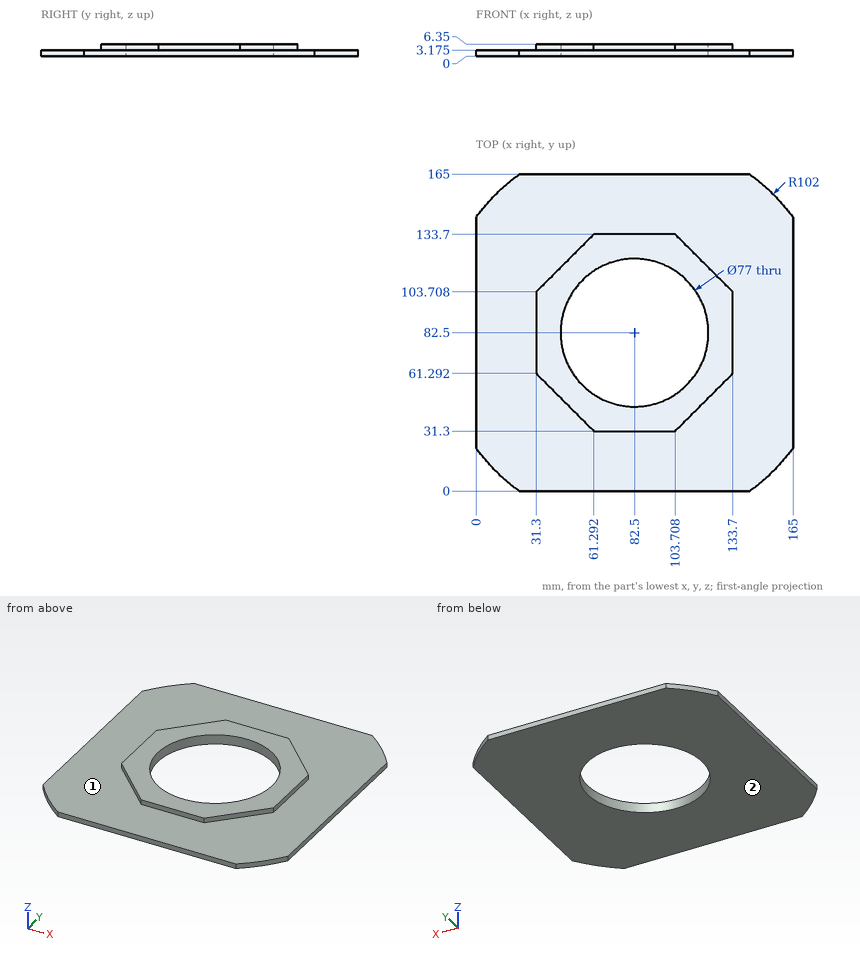
Drawing for the job (mm, zero at the part's lowest x, y, z). A direction names the side the tool comes from. Round coordinates to 2 decimals unless told otherwise and drop trailing zeros. Answer in a Markdown table with one row per item.
Item 1: Drill centre lines: L1, parallel to Y at x = 82.5, z = 1.5; L2, parallel to Y at x = 82.5, z = 5.25; L3, parallel to Z at x = 27.5, y = 34 (1 decimal). Where is each one in solid material? Low to high. Write a range as [from, to].
Answers below:
| item | result |
|---|---|
| L1 | y = [0, 44], [121, 165] |
| L2 | y = [31.3, 44], [121, 133.7] |
| L3 | z = [0, 3.2] |
Item 2: Which spindle directions (+Z, -Z, +X, -X, +Y, -Y) get a long thin tool onto all of the face, cutting with end or side? Do the marked faces 1 and 2. Say none if no direction does.
Answers below:
| item | result |
|---|---|
| face 1 | +Z |
| face 2 | -Z, +X, -X, +Y, -Y |
Item 3: Pin check, flat tips, straight feed: pin 1 (2.5 mm diameter, centred on y = 76.5, z = 5, fed in from +X); pin 2 (1 mm diameter, centred on x = 82.5, z = 4.5, fed in from -Y); pin 3 (1.5 mm diameter, centred on y = 115.5, z = 3.5, fed in from -X); pin 4 (10 mm diameter, centred on x = 127.5, y = 37.5, fed in from +Z) (3 decimals). Stop position of each tip, or through.
Answers below:
| item | result |
|---|---|
| pin 1 | stops at x = 133.7 |
| pin 2 | stops at y = 31.3 |
| pin 3 | stops at x = 0 |
| pin 4 | stops at z = 3.175 |
